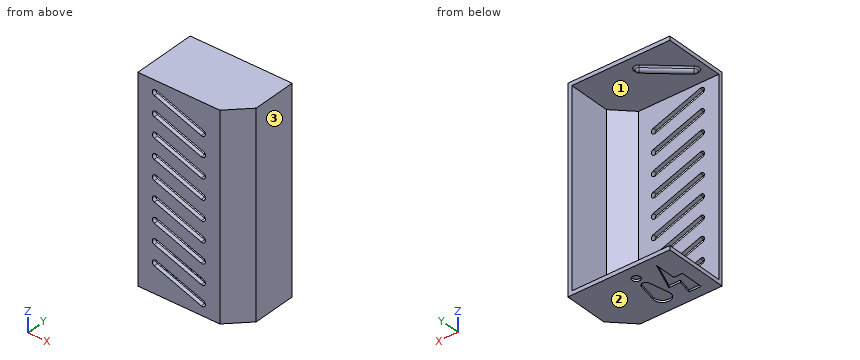
```python
from build123d import *

# Parameters (mm, degrees)
BOSS_EXTRUDE1_DEPTH = 30
SKETCH3_W           = 50.97
SKETCH3_H           = 100.4
BOSS_EXTRUDE2_DEPTH = 2
REVOLVE1_ANGLE      = 358
FILLET1_R           = 1
CUT_EXTRUDE1_DEPTH  = 101
BOSS_EXTRUDE3_REACH = 170.96
CUT_EXTRUDE2_DEPTH  = 2
LPATTERN1_COUNT     = 5
LPATTERN1_PITCH     = 10
LPATTERN2_COUNT     = 5
LPATTERN2_PITCH     = 10
SKETCH9_R           = 2
SKETCH9_R_2         = 4
CUT_EXTRUDE3_DEPTH  = 1


with BuildPart() as part:
    # Sketch2 → Boss-Extrude1 (new body)
    with BuildSketch(Plane.XZ.offset(30)):
        Polygon((-133.57, -96.2), (-84.6, -96.2), (-84.6, 0.2), (-133.57, 0.2), (-133.57, 2.2), (-82.6, 2.2), (-82.6, -98.2), (-133.57, -98.2), align=None)
    extrude(amount=-BOSS_EXTRUDE1_DEPTH)

    # Sketch3 → Boss-Extrude2 (add)
    with BuildSketch(Plane.XZ.offset(30)):
        with Locations((-108.085, -48)):
            Rectangle(SKETCH3_W, SKETCH3_H)
    extrude(amount=BOSS_EXTRUDE2_DEPTH)

    # Sketch4 → Revolve1 (revolve)
    with BuildSketch(Plane(origin=(0, 0, 0.2), x_dir=(-1, 0, 0), z_dir=(0, 0, -1))):
        with BuildLine():
            ThreePointArc((126.946389188, -22.830754007), (128.214647144, -23.261442668), (129.415983818, -22.669191741))
            Line((129.415983818, -22.669191741), (110.772864663, -6.315578448))
            ThreePointArc((110.772864663, -6.315578448), (110.342176002, -7.583836403), (110.934426929, -8.785173077))
            Line((110.934426929, -8.785173077), (126.946389188, -22.830754007))
        make_face()
    revolve1 = revolve(axis=Axis((-128.10040537, -21.515175559, 0.2), (0.7517591128712743, 0.6594378183081363, 0)), revolution_arc=REVOLVE1_ANGLE)

    # Mirror3: Revolve1 across plane
    add(revolve1.mirror(Plane(origin=(0, 0, -48), x_dir=(1, 0, 0), z_dir=(0, 0, -1))))

    # Fillet1
    fillet1_edges = [part.edges().sort_by_distance(p)[0] for p in [
        (-128.214647144, -23.261442668, 0.2),
        (-121.248440423, -13.176806647, 0.2),
        (-111.974201337, -5.72332752, 0.2),
        (-118.940408059, -15.807963542, 0.2),
        (-128.214647144, -23.261442668, -96.2),
        (-121.248440423, -13.176806647, -96.2),
        (-111.974201337, -5.72332752, -96.2),
        (-118.940408059, -15.807963542, -96.2),
    ]]
    fillet(fillet1_edges, radius=FILLET1_R)

    # Sketch5 → Cut-Extrude1 (cut)
    with BuildSketch(Plane(origin=(0, 0, -98.2), x_dir=(-1, 0, 0), z_dir=(0, 0, -1))):
        Polygon((92.6, -32), (82.6, -22), (82.6, -32), align=None)
    extrude(amount=-CUT_EXTRUDE1_DEPTH, mode=Mode.SUBTRACT)

    # Sketch7 → Boss-Extrude3 (add, up to next)
    with BuildSketch(Plane(origin=(0, 0, 0.2), x_dir=(-1, 0, 0), z_dir=(0, 0, -1)), mode=Mode.PRIVATE) as boss_extrude3_sk1:
        Polygon((93.428427125, -30), (84.6, -21.171572875), (84.6, -24), (90.6, -30), align=None)
    boss_extrude3_tool1 = extrude(boss_extrude3_sk1.sketch, amount=BOSS_EXTRUDE3_REACH, mode=Mode.PRIVATE) - part.part
    add(boss_extrude3_tool1.solids().sort_by_distance((-88.352065, -26.247935, 0.2))[0])

    # Sketch8 → Cut-Extrude2 (cut)
    with BuildSketch(Plane.XZ.offset(32)):
        with BuildLine():
            Line((-101.851872455, -53.684790723), (-125.344187975, -45.13428714))
            ThreePointArc((-125.344187975, -45.13428714), (-126.240696691, -43.211717993), (-124.318127545, -42.315209277))
            Line((-124.318127545, -42.315209277), (-100.825812025, -50.86571286))
            ThreePointArc((-100.825812025, -50.86571286), (-99.929303309, -52.788282007), (-101.851872455, -53.684790723))
        make_face()
    cut_extrude2 = extrude(amount=-CUT_EXTRUDE2_DEPTH, mode=Mode.SUBTRACT)

    # LPattern1: Cut-Extrude2 ×5
    with Locations(*[(0, 0, -i * LPATTERN1_PITCH) for i in range(1, LPATTERN1_COUNT)]):
        add(cut_extrude2, mode=Mode.SUBTRACT)

    # LPattern2: Cut-Extrude2 ×5
    with Locations(*[(0, 0, i * LPATTERN2_PITCH) for i in range(1, LPATTERN2_COUNT)]):
        add(cut_extrude2, mode=Mode.SUBTRACT)

    # Sketch9 → Cut-Extrude3 (cut)
    with BuildSketch(Plane(origin=(0, 0, -98.2), x_dir=(-1, 0, 0), z_dir=(0, 0, -1))):
        with Locations((111.05096655, -7)):
            Circle(SKETCH9_R)
        with Locations((111.05096655, -23)):
            Circle(SKETCH9_R_2)
        with Locations((111.05096655, -13)):
            Circle(SKETCH9_R)
        Polygon((127.147055737, -27), (121.090407141, -27), (122.676520454, -19.790973413), (116.946384418, -19.790973413), (122.811770426, -5), (122.811770426, -15.583196494), (127.147055737, -15.583196494), align=None)
        Polygon((113.010558344, -12.6), (114.970150138, -22.2), (107.131782961, -22.2), (109.091374756, -12.6), align=None)
    extrude(amount=-CUT_EXTRUDE3_DEPTH, mode=Mode.SUBTRACT)


solid = part.part
```
Geometry: final body of the model. Coordinates: model frame, mm. Face numbers are marked on the shaded views. Coordinates: 2 decimals unless noted, no trailing zeros. Use a Markdown table: item, result. Add a question column.
(1) Pin query (flat end, axial travel): pin 1 Ø12 at (x, z) = (-116.5, -17.5) entering from +Y; pin 2 Ø1.5 at (x, y) = (-112, -17.5) entering from -Z; pin 3 Ø3 at (y, z) = (-26, -8.5) entering from -X. Return the tip coordinate at first contact, or that it passes through.
(2) Line query: line 1 along Z through (x, y) = (-110, -3); line 2 along Z through (x, y) = (-127, -16); line 3 along X through (y, z) = (-8.5, -11). Output: solid intervals per line, ascending.
(3) Mould query, pull axis X, two halves, no side actions, for the marked faces 1, 2 and 3. Classes: pulls with the +X half, pulls with the -X half, needs draft (parallel to the pull), parting line crosses it, or undercut.
Answer:
| question | item | result |
|---|---|---|
| 1 | pin 1 | stops at y = -30 |
| 1 | pin 2 | stops at z = -97.2 |
| 1 | pin 3 | stops at x = -90.93 |
| 2 | line 1 | z = -98.2 to -96.2, 0.2 to 2.2 |
| 2 | line 2 | z = -97.2 to -96.2, 0.2 to 2.2 |
| 2 | line 3 | x = -84.6 to -82.6 |
| 3 | face 1 | undercut |
| 3 | face 2 | needs draft |
| 3 | face 3 | pulls with the +X half |
